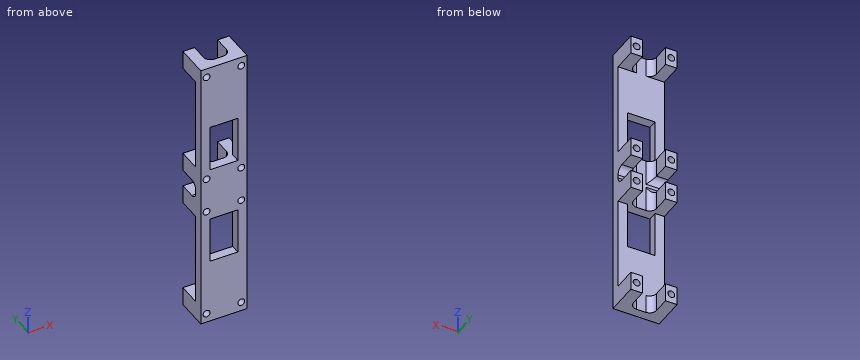
Autodesk Inventor part; units mm, degrees
ref_plane "YZ Plane" through (0, 0, 0) normal (1, 0, 0) x (0, 1, 0)
ref_plane "XZ Plane" through (0, 0, 0) normal (0, 1, 0) x (-1, 0, 0)
ref_plane "XY Plane" through (0, 0, 0) normal (0, 0, 1) x (1, 0, 0)
sketch "Sketch1" plane through (0, 0, 0) normal (0, 1, 0) x (-1, 0, 0)
  line L0 (0, 0) -> (20, 0)
  line L1 (20, 0) -> (20, -120)
  line L2 (20, -120) -> (0, -120)
  line L3 (0, -120) -> (0, 0)
  dimension "d0" = 20
  dimension "d1" = 120
extrude "Extrusion1" add sketch "Sketch1" along normal blind 4
sketch "Sketch2" plane through (0, 4, 0) normal (0, 1, 0) x (1, 0, 0)
  line L0 (-20, 0) -> (0, 0)
  line L1 (0, 0) -> (0, 120)
  line L2 (-20, 0) -> (0, 0)
  line L3 (0, 0) -> (0, 8)
  line L4 (0, 8) -> (-20, 8)
  line L5 (-20, 8) -> (-20, 0)
  line L6 (-20, 8) -> (0, 8)
  line L7 (0, 8) -> (0, 48.3)
  line L8 (0, 48.3) -> (-20, 48.3)
  line L9 (-20, 48.3) -> (-20, 8)
  line L10 (-20, 48.3) -> (0, 48.3)
  line L11 (0, 48.3) -> (0, 56.3)
  line L12 (0, 56.3) -> (-20, 56.3)
  line L13 (-20, 56.3) -> (-20, 48.3)
  line L14 (-20, 120) -> (-20, 0)
  line L15 (-20, 120) -> (0, 120)
  line L16 (0, 120) -> (0, 112)
  line L17 (0, 112) -> (-20, 112)
  line L18 (-20, 112) -> (-20, 120)
  line L19 (-20, 112) -> (0, 112)
  line L20 (0, 112) -> (0, 71.7)
  line L21 (0, 71.7) -> (-20, 71.7)
  line L22 (-20, 71.7) -> (-20, 112)
  line L23 (-20, 71.7) -> (0, 71.7)
  line L24 (0, 71.7) -> (0, 63.7)
  line L25 (0, 63.7) -> (-20, 63.7)
  line L26 (-20, 63.7) -> (-20, 71.7)
  line L27 (-20, 0) -> (-15, 0)
  line L28 (-15, 0) -> (-15, 8)
  line L29 (-15, 8) -> (-20, 8)
  line L30 (-20, 8) -> (-20, 0)
  line L31 (0, 8) -> (-5, 8)
  line L32 (-5, 8) -> (-5, 0)
  line L33 (-5, 0) -> (0, 0)
  line L34 (0, 0) -> (0, 8)
  line L35 (-20, 48.3) -> (-15, 48.3)
  line L36 (-15, 48.3) -> (-15, 56.3)
  line L37 (-15, 56.3) -> (-20, 56.3)
  line L38 (-20, 56.3) -> (-20, 48.3)
  line L39 (0, 48.3) -> (-5, 48.3)
  line L40 (-5, 48.3) -> (-5, 56.3)
  line L41 (-5, 56.3) -> (0, 56.3)
  line L42 (0, 56.3) -> (0, 48.3)
  line L43 (-20, 63.7) -> (-15, 63.7)
  line L44 (-15, 63.7) -> (-15, 71.7)
  line L45 (-15, 71.7) -> (-20, 71.7)
  line L46 (-20, 71.7) -> (-20, 63.7)
  line L47 (0, 63.7) -> (-5, 63.7)
  line L48 (-5, 63.7) -> (-5, 71.7)
  line L49 (-5, 71.7) -> (0, 71.7)
  line L50 (0, 71.7) -> (0, 63.7)
  line L51 (-20, 112) -> (-15, 112)
  line L52 (-15, 112) -> (-15, 120)
  line L53 (-15, 120) -> (-20, 120)
  line L54 (-20, 120) -> (-20, 112)
  line L55 (0, 112) -> (-5, 112)
  line L56 (-5, 112) -> (-5, 120)
  line L57 (-5, 120) -> (0, 120)
  line L58 (0, 120) -> (0, 112)
  dimension "d4" = 8
  dimension "d5" = 40.3
  dimension "d6" = 8
  dimension "d7" = 20
  dimension "d8" = 8
  dimension "d9" = 40.3
  dimension "d10" = 8
  dimension "d11" = 5
  dimension "d12" = 5
  dimension "d13" = 8
  dimension "d14" = 5
  dimension "d15" = 5
  dimension "d16" = 5
  dimension "d17" = 5
  dimension "d18" = 5
  dimension "d19" = 5
extrude "Extrusion2" add sketch "Sketch2" along normal blind 10 contours L5 L4 L28 L0 | L32 L4 L1 L0 | L13 L12 L36 L8 | L40 L12 L1 L8 | L14 L21 L44 L25 | L14 L15 L52 L17 | L48 L21 L1 L25 | L56 L15 L1 L17
sketch "Sketch3" plane through (0, 14, 0) normal (0, 1, 0) x (1, 0, 0)
  line L0 (-20, 120) -> (-20, 0)
  line L1 (-20, 0) -> (-17.5, 0)
  line L2 (-17.5, 0) -> (-17.5, 4)
  line L3 (-17.5, 4) -> (-20, 4)
  line L4 (-20, 4) -> (-20, 0)
  line L5 (0, 0) -> (0, 120)
  line L6 (0, 0) -> (-2.5, 0)
  line L7 (-2.5, 0) -> (-2.5, 4)
  line L8 (-2.5, 4) -> (0, 4)
  line L9 (0, 4) -> (0, 0)
  line L10 (-15, 56.3) -> (-20, 56.3)
  line L11 (-20, 56.3) -> (-17.5, 56.3)
  line L12 (-17.5, 56.3) -> (-17.5, 52.3)
  line L13 (-17.5, 52.3) -> (-20, 52.3)
  line L14 (-20, 52.3) -> (-20, 56.3)
  line L15 (-5, 56.3) -> (0, 56.3)
  line L16 (-5, 56.3) -> (-2.5, 56.3)
  line L17 (-2.5, 56.3) -> (-2.5, 52.3)
  line L18 (-2.5, 52.3) -> (-5, 52.3)
  line L19 (-5, 52.3) -> (-5, 56.3)
  line L20 (-20, 120) -> (-17.5, 120)
  line L21 (-17.5, 120) -> (-17.5, 116)
  line L22 (-17.5, 116) -> (-20, 116)
  line L23 (-20, 116) -> (-20, 120)
  line L24 (-5, 120) -> (-2.5, 120)
  line L25 (-2.5, 120) -> (-2.5, 116)
  line L26 (-2.5, 116) -> (-5, 116)
  line L27 (-5, 116) -> (-5, 120)
  line L28 (-20, 71.7) -> (-15, 71.7)
  line L29 (-15, 71.7) -> (-17.5, 71.7)
  line L30 (-17.5, 71.7) -> (-17.5, 67.7)
  line L31 (-17.5, 67.7) -> (-15, 67.7)
  line L32 (-15, 67.7) -> (-15, 71.7)
  line L33 (-5, 71.7) -> (-2.5, 71.7)
  line L34 (-2.5, 71.7) -> (-2.5, 67.7)
  line L35 (-2.5, 67.7) -> (-5, 67.7)
  line L36 (-5, 67.7) -> (-5, 71.7)
  circle A0 centre (-17.5, 67.7) radius 1.5
  circle A1 centre (-2.5, 67.7) radius 1.5
  circle A2 centre (-17.5, 116) radius 1.5
  circle A3 centre (-2.5, 116) radius 1.5
  circle A4 centre (-17.5, 52.3) radius 1.5
  circle A5 centre (-2.5, 52.3) radius 1.5
  circle A6 centre (-17.5, 4) radius 1.5
  circle A7 centre (-2.5, 4) radius 1.5
  dimension "d22" = 2.5
  dimension "d23" = 4
  dimension "d24" = 2.5
  dimension "d25" = 4
  dimension "d26" = 2.5
  dimension "d27" = 4
  dimension "d28" = 2.5
  dimension "d29" = 4
  dimension "d30" = 2.5
  dimension "d31" = 4
  dimension "d32" = 2.5
  dimension "d33" = 4
  dimension "d34" = 2.5
  dimension "d35" = 4
  dimension "d36" = 2.5
  dimension "d37" = 4
  dimension "d38" = 3
  dimension "d39" = 3
  dimension "d40" = 3
  dimension "d41" = 3
  dimension "d42" = 3
  dimension "d43" = 3
  dimension "d44" = 3
  dimension "d45" = 3
extrude "Extrusion3" cut sketch "Sketch3" against normal up to surface (14 mm away) contours A2 L21 L22 | L22 L21 A2 | A0 L31 L30 | L30 L31 A0 | A4 L12 L13 | L13 L12 A4 | A6 L2 L3 | L3 L2 A6 | A7 L7 L8 | L8 L7 A7 | A5 L18 L17 | L17 L18 A5 | A3 L26 L25 | L25 L26 A3 | A1 L35 L34 | L34 L35 A1
fillet "Fillet1" radius 3 12 edges at (-15, 4, -52.3) (-5, 4, -52.3) (-15, 4, -67.7) (-17.5, 4, -63.7) (-17.5, 4, -56.3) (-2.5, 4, -63.7) (-2.5, 4, -56.3) (-5, 4, -67.7) (-15, 4, -4) (-5, 4, -4) (-15, 4, -116) (-5, 4, -116)
sketch "Sketch5" plane through (0, 4, 0) normal (0, 1, 0) x (1, 0, 0)
  line L0 (0, 48.3) -> (-8, 48.3)
  line L1 (0, 48.3) -> (-4, 48.3)
  line L2 (-8, 71.7) -> (0, 71.7)
  line L3 (0, 71.7) -> (-4, 71.7)
  line L4 (-4, 71.7) -> (-16, 71.7)
  line L5 (-16, 71.7) -> (-16, 91.7)
  line L6 (-16, 91.7) -> (-4, 91.7)
  line L7 (-4, 91.7) -> (-4, 71.7)
  line L8 (-4, 48.3) -> (-16, 48.3)
  line L9 (-16, 48.3) -> (-16, 28.3)
  line L10 (-16, 28.3) -> (-4, 28.3)
  line L11 (-4, 28.3) -> (-4, 48.3)
  point P0 (0, 0)
  dimension "d63" = 4
  dimension "d64" = 4
  dimension "d65" = 12
  dimension "d66" = 20
  dimension "d67" = 12
  dimension "d68" = 20
extrude "Extrusion5" cut sketch "Sketch5" against normal blind 8
sketch "Sketch6" plane through (0, 0, 0) normal (0, -1, 0) x (1, 0, 0)
  circle A0 centre (-2.5, -4) radius 1.5
  circle A1 centre (-2.5, -4) radius 4
  circle A2 centre (-17.5, -4) radius 1.5
  circle A3 centre (-17.5, -4) radius 4
  circle A4 centre (-17.5, -52.3) radius 1.5
  circle A5 centre (-17.5, -52.3) radius 4
  circle A6 centre (-2.5, -52.3) radius 1.5
  circle A7 centre (-2.5, -52.3) radius 4
  circle A8 centre (-17.5, -67.7) radius 1.5
  circle A9 centre (-17.5, -67.7) radius 4
  circle A10 centre (-2.5, -67.7) radius 1.5
  circle A11 centre (-2.5, -67.7) radius 4
  circle A12 centre (-17.5, -116) radius 1.5
  circle A13 centre (-17.5, -116) radius 4
  circle A14 centre (-2.5, -116) radius 1.5
  circle A15 centre (-2.5, -116) radius 4
  line L0 (0, -120) -> (-20, -120)
  line L1 (-20, -120) -> (-17.5, -120)
  line L2 (-17.5, -120) -> (-17.5, -116)
  line L3 (-17.5, -116) -> (-20, -116)
  line L4 (-20, -116) -> (-20, -120)
  line L5 (0, -120) -> (-2.5, -120)
  line L6 (-2.5, -120) -> (-2.5, -116)
  line L7 (-2.5, -116) -> (0, -116)
  line L8 (0, -116) -> (0, -120)
  line L9 (-20, -120) -> (-20, 0)
  line L10 (-20, 0) -> (-17.5, 0)
  line L11 (-17.5, 0) -> (-17.5, -4)
  line L12 (-17.5, -4) -> (-20, -4)
  line L13 (-20, -4) -> (-20, 0)
  line L14 (0, 0) -> (-2.5, 0)
  line L15 (-2.5, 0) -> (-2.5, -4)
  line L16 (-2.5, -4) -> (0, -4)
  line L17 (0, -4) -> (0, 0)
  dimension "d71" = 8
  dimension "d72" = 8
  dimension "d73" = 8
  dimension "d74" = 8
  dimension "d75" = 8
  dimension "d76" = 8
  dimension "d77" = 8
properties part number "support_2_servos"
Part model, mm, in its own coordinate system. Round coordinates to 2 decimals unless told otherwise and drop trailing zeros. Write each loop counter-clockwise with the first axis right and the second up, starting at its lowest first coordinate (ties: lowest second). Pieces come first, ordered by that corner, then holes. Notation, with made-up numbers: M 77,17.25 L 122,17.25 A20 cw 122,41.25 Z; hole C 69,33.25 d3. An arc over 180 degrees is marked long. Answer as CSV lines item,"result". Start each with the question number.
1) Drop flat-ended pins along their axis: pin 1 (3 mm diameter, centred on y = 2.5, z = -80, fed in from +X); pin 2 (1 mm diameter, centred on x = -17, z = -39, fed in from +Y); pin 3 (4 mm diameter, centred on x = -11, z = -74.5, fed in from +Y). Give the stop position or say it passes through.
2) Band-saw the part on B-B (x = -2.5). Count the separate pieces of the cut face and the enclosed holes in it, then the cut area to 3 significant figures.
3) Drill centre lines: L1, parallel to X at y = 9.5, z = -52.3; L2, parallel to Z at x = -6.5, y = 2.25; L3, parallel to Z at x = -2.5, y = 3.5. Where is each one in solid material? Low to high.
4) Band-saw the part on D-D (x = -10.25). List the corners of the cut face in (y, z), then the cut area to 3 significant figures.
5) Band-saw the part on A-A (z = -4). List the corners of the cut face in (x, y).
Worked out:
1,pin 1,"x = 0"
1,pin 2,"y = 4"
1,pin 3,"through"
2,separate pieces,"5"
2,enclosed holes,"0"
2,area,"636 mm²"
3,L1,"-20 to -19, -16 to -15, -5 to -4, -1 to 0"
3,L2,"-120 to -91.7, -71.7 to -48.3, -28.3 to 0"
3,L3,"-120 to -117.5, -114.5 to -69.2, -66.2 to -53.8, -50.8 to -5.5, -2.5 to 0"
4,outline,"M 0,-120 L 4,-120 L 4,-91.7 L 0,-91.7 Z; M 0,-71.7 L 4,-71.7 L 4,-48.3 L 0,-48.3 Z; M 0,-28.3 L 4,-28.3 L 4,0 L 0,0 Z"
4,area,"320 mm²"
5,outline,"M -20,0 L -19,0 L -19,14 L -20,14 Z; M -16,0 L -4,0 L -4,14 L -5,14 L -5,7 A3 cw -8,4 L -12,4 A3 cw -15,7 L -15,14 L -16,14 Z; M -1,0 L 0,0 L 0,14 L -1,14 Z"
